from build123d import *

# Parameters (mm, degrees)
F0_R     = 1.7145
F0_W     = 7.9375
F0_H     = 3.175
F1_DEPTH = 3.175
F3_DEPTH = 3.176
F4_R     = 5.08


with BuildPart() as f1:
    # F0 (on Top) → F1 (new body)
    with BuildSketch(Plane.XY):
        Polygon((-142.08125, 101.6), (-188.9125, -101.6), (188.9125, -101.6), (142.08125, 101.6), align=None)
        Polygon((-172.0488805663, -65.1862989442), (-175.1427761754, -64.4732526906), (-173.3601605412, -56.7385136678), (-170.2662649321, -57.4515599214), align=None, mode=Mode.SUBTRACT)
        with Locations((-169.6740739757, -47.8133499672)):
            Circle(F0_R, mode=Mode.SUBTRACT)
        Polygon((-169.0818830192, -38.175140013), (-167.2992673851, -30.4404009902), (-164.205371776, -31.1534472439), (-165.9879874101, -38.8881862667), align=None, mode=Mode.SUBTRACT)
        Polygon((172.0488805663, -65.1862989442), (170.2662649321, -57.4515599214), (173.3601605412, -56.7385136678), (175.1427761754, -64.4732526906), align=None, mode=Mode.SUBTRACT)
        with Locations((169.6740739757, -47.8133499672)):
            Circle(F0_R, mode=Mode.SUBTRACT)
        Polygon((167.2992673851, -30.4404009902), (169.0818830192, -38.175140013), (165.9879874101, -38.8881862667), (164.205371776, -31.1534472439), align=None, mode=Mode.SUBTRACT)
        Polygon((-150.0182030992, 30.4044371841), (-151.8008187334, 22.6696981613), (-154.8947143425, 23.3827444149), (-153.1120987083, 31.1174834377), align=None, mode=Mode.SUBTRACT)
        with Locations((-149.5820584881, 39.7220878176)):
            Circle(F0_R, mode=Mode.SUBTRACT)
        Polygon((-145.8959719225, 48.2907283913), (-148.9898675317, 49.003774645), (-147.2072518975, 56.7385136678), (-144.1133562884, 56.0254674141), align=None, mode=Mode.SUBTRACT)
        with Locations((-69.85, 94.0125)):
            Rectangle(F0_W, F0_H, mode=Mode.SUBTRACT)
        Polygon((150.0182030992, 30.4044371841), (153.1120987083, 31.1174834377), (154.8947143425, 23.3827444149), (151.8008187334, 22.6696981613), align=None, mode=Mode.SUBTRACT)
        with Locations((149.5820584881, 39.7220878176)):
            Circle(F0_R, mode=Mode.SUBTRACT)
        with Locations((69.85, 94.0125)):
            Rectangle(F0_W, F0_H, mode=Mode.SUBTRACT)
        Polygon((145.8959719225, 48.2907283913), (144.1133562884, 56.0254674141), (147.2072518975, 56.7385136678), (148.9898675317, 49.003774645), align=None, mode=Mode.SUBTRACT)
    extrude(amount=F1_DEPTH)

    # F2 (on face) → F3 (cut, through all)
    with BuildSketch(Plane.XY.offset(3.175)):
        Polygon((0, 80.9625), (-100.0125, 80.9625), (-100.0125, 36.5125), (-49.2125, 36.5125), (-49.2125, -101.6), (0, -101.6), (49.2125, -101.6), (49.2125, 36.5125), (100.0125, 36.5125), (100.0125, 80.9625), align=None)
    extrude(amount=-F3_DEPTH, mode=Mode.SUBTRACT)

    # F4
    f4_edges = [f1.edges().sort_by_distance(p)[0] for p in [
        (-142.08125, 101.6, 1.5875),
        (-188.9125, -101.6, 1.5875),
        (142.08125, 101.6, 1.5875),
        (188.9125, -101.6, 1.5875),
        (-49.2125, -101.6, 1.5875),
        (49.2125, -101.6, 1.5875),
        (-100.0125, 80.9625, 1.5875),
        (-49.2125, 36.5125, 1.5875),
        (-100.0125, 36.5125, 1.5875),
        (49.2125, 36.5125, 1.5875),
        (100.0125, 80.9625, 1.5875),
        (100.0125, 36.5125, 1.5875),
    ]]
    fillet(f4_edges, radius=F4_R)


solid = f1.part
Geometry: final body of the model. Coordinates: model frame, mm. Give positions to 0.01 mm unless a question says otherwise; leave off trailing zeros. Loops run counter-clockwise (first coordinate to the right, second up) from the corner with the lowest first, then second, coordinate; pieces in that order, holes last. Notation, with made-up numbers: (5.25, 67) - (52.25, 67) arc R18 cw to (52.25, 80) - close; hole circle Ø5 at (27.5, 68). An arc over 180 degrees is marked (long way). Answer as CSV lines item,"result". Start each with the question number.
1. Pin query (flat end, axial travel): P1, Ø2.5, axis at x = 169.67, y = -47.81, coming from the +Z side; P2, Ø1, axis at y = 94.5, z = 1.5, coming from the +X side; P3, Ø1.6, axis at y = 93.5, z = 2, coming from the -X side; P4, Ø5, axis at x = 121.5, y = 56.5, coming from the -Z side. Return the tip coordinate at first contact, or that it passes through.
2. Section A-A, the plane y = 68. Return loops of the section in (x, z) (1 decimal), plus the area to 3 significant figures.
3. Section B-B, the plane x = 6. Return loops of the section in (y, z) (1 decimal).
4. Section C-C, the plane z = 2.45. Give the number of separate pieces and of enclosed holes in the cut face, plus the area to 3 significant figures.
5. Ray query, L1, parallel to Y at x = 74, z = 0.3; L2, parallel to X at y = -74, z = 1; L3, parallel to X at y = -2, z = 2.25. Return the intervals inside material, ascending.
Answers:
1,P1,"passes through"
1,P2,"stops at x = 143.83"
1,P3,"stops at x = -144.13"
1,P4,"stops at z = 0"
2,outline,"(-149.8, 0) - (-100, 0) - (-100, 3.2) - (-149.8, 3.2) - close; (100, 0) - (149.8, 0) - (149.8, 3.2) - (100, 3.2) - close"
2,area,"316 mm2"
3,outline,"(81, 0) - (101.6, 0) - (101.6, 3.2) - (81, 3.2) - close"
4,separate pieces,"1"
4,enclosed holes,"14"
4,area,"44,500 mm2"
5,L1,"y = -101.6 to 36.51, 80.96 to 101.6"
5,L2,"x = -182.55 to -49.21, 49.21 to 182.55"
5,L3,"x = -165.96 to -49.21, 49.21 to 165.96"
